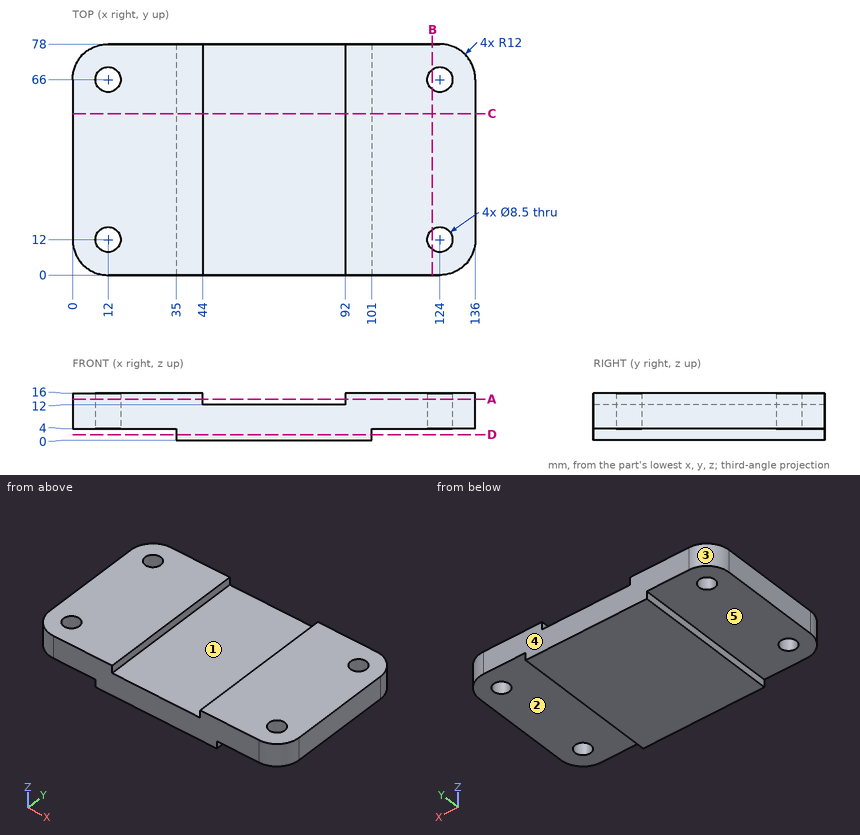
The figure shows three views and two pictorial views of one solid part (mm, origin at its lowest corner). Answer the questions. A direction names the side the tool comes from. Coordinates: 2 decimals unless noted, no trailing zeros. Write each loop counter-clockwise with the first axis right and the second up, starting at its lowest first coordinate (ties: lowest second). Pieces come first, ordered by that corner, then holes. Notation, with made-up numbers: (36, 78.25) -> (65, 78.25) arc R28 ccw to (65, 98.25) -> close; hole circle Ø7 at (-13, -39.5). An arc over 180 degrees is marked (long way). Return JSON: item names as keys, results as strings.
(1) For a pull along X with two mould halves and no side action, classify the marked faces 1, 2 and 3 as pulls with the +X half, pulls with the -X half, needs draft (parallel to the pull), parting line crosses it, or undercut.
Answers below:
{"face 1": "undercut", "face 2": "needs draft", "face 3": "pulls with the -X half"}
(2) The part is cut by section D-D on z = 2. Give the vertices of the cut face in (x, y), then the cut area to 3 significant figures.
Answers below:
{"outline": "(35, 0) -> (101, 0) -> (101, 78) -> (35, 78) -> close", "area": "5,150 mm^2"}
(3) Consider line 1 along X through (y, z) = (66.5, 12.25); line 2 along Y through (x, z) = (12, 10); line 3 along X through (y, z) = (30, 15). Determine where each line is inside the solid, lowest interval first. Write a range as from..to.
Answers below:
{"line 1": "0.01..7.78, 16.22..44, 92..119.78, 128.22..135.99", "line 2": "0..7.75, 16.25..61.75, 70.25..78", "line 3": "0..44, 92..136"}
(4) The part is cut by section B-B on x = 121.5. Give the vertices of the cut face in (y, z).
Answers below:
{"outline": "(0, 4) -> (8.56, 4) -> (8.56, 16) -> (0, 16) -> close; (15.44, 4) -> (62.56, 4) -> (62.56, 16) -> (15.44, 16) -> close; (69.44, 4) -> (78, 4) -> (78, 16) -> (69.44, 16) -> close"}
(5) The part is cut by section A-A on z = 14. Give the vertices of the cut face in (x, y), then the cut area to 3 significant figures.
Answers below:
{"outline": "(0, 12) arc R12 ccw to (12, 0) -> (44, 0) -> (44, 78) -> (12, 78) arc R12 ccw to (0, 66) -> close; (92, 0) -> (124, 0) arc R12 ccw to (136, 12) -> (136, 66) arc R12 ccw to (124, 78) -> (92, 78) -> close; hole circle Ø8.5 at (12, 12); hole circle Ø8.5 at (12, 66); hole circle Ø8.5 at (124, 12); hole circle Ø8.5 at (124, 66)", "area": "6,510 mm^2"}
(6) Which of the six approach directions +Z, -Z, +X, -X, +Y, -Y give full straight-line access (tool end or side, diameter ignored) to the marked faces 4 and 5?
Answers below:
{"face 4": "+Z, -Z, +X, -X, +Y", "face 5": "-Z, -X, +Y, -Y"}
(7) Each of these flat-tipped pins is pushed along its axis until it touches: P1, Ø5, axis at x = 124, y = 12, coming from the -Z side; P2, Ø4.5, axis at y = 55, z = 1.5, coming from the -X side; P3, Ø5, axis at y = 67, z = 3.5, coming from the +X side; P4, Ø14.5, axis at x = 74.5, y = 23.5, coming from the +Z side. Where does it stop, or does it pass through?
Answers below:
{"P1": "through", "P2": "x = 35", "P3": "x = 136", "P4": "z = 12"}
(8) The part is cut by section C-C on y = 54.5. Give the vertices of the cut face in (x, z), then the cut area to 3 significant figures.
Answers below:
{"outline": "(0, 4) -> (35, 4) -> (35, 0) -> (101, 0) -> (101, 4) -> (136, 4) -> (136, 16) -> (92, 16) -> (92, 12) -> (44, 12) -> (44, 16) -> (0, 16) -> close", "area": "1,700 mm^2"}
